```python
from build123d import *

# Parameters (mm, degrees)
SKETCH1_R               = 25
BOSS_EXTRUDE1_DEPTH     = 5
SKETCH3_R               = 1
CUT_EXTRUDE2_DEPTH      = 6
SKETCH4_R               = 25
SKETCH4_R_2             = 20.666666667
BOSS_EXTRUDE2_DEPTH     = 12
SKETCH2_R               = 1.3
CUT_EXTRUDE1_DEPTH      = 13
CUT_EXTRUDE1_DEPTH_BACK = 6
CUT_EXTRUDE3_DEPTH      = 6
CUT_EXTRUDE5_DEPTH      = 13
SKETCH8_R               = 2.3
SKETCH8_R_2             = 1.3
BOSS_EXTRUDE3_DEPTH     = 12


with BuildPart() as part:
    # Sketch1 → Boss-Extrude1 (new body)
    with BuildSketch(Plane(origin=(0, 0, 0), x_dir=(0, 0, -1), z_dir=(1, 0, 0))):
        Circle(SKETCH1_R)
    extrude(amount=BOSS_EXTRUDE1_DEPTH)

    # Sketch3 → Cut-Extrude2 (cut, through all)
    with BuildSketch(Plane.ZY):
        with Locations((-13.14, 13.14)):
            Circle(SKETCH3_R)
        with Locations((13.14, 13.14)):
            Circle(SKETCH3_R)
        with Locations((13.14, -13.14)):
            Circle(SKETCH3_R)
        with Locations((-13.14, -13.14)):
            Circle(SKETCH3_R)
    extrude(amount=-CUT_EXTRUDE2_DEPTH, mode=Mode.SUBTRACT)

    # Sketch4 → Boss-Extrude2 (add)
    with BuildSketch(Plane(origin=(5, 0, 0), x_dir=(0, 0, -1), z_dir=(1, 0, 0))):
        Circle(SKETCH4_R)
        Circle(SKETCH4_R_2, mode=Mode.SUBTRACT)
    extrude(amount=BOSS_EXTRUDE2_DEPTH)

    # Sketch2 → Cut-Extrude1 (cut, two sides)
    with BuildSketch(Plane(origin=(5, 0, 0), x_dir=(0, 0, -1), z_dir=(1, 0, 0))) as cut_extrude1_sk:
        with Locations((0, 21.5)):
            Circle(SKETCH2_R)
        with Locations((21.5, 0)):
            Circle(SKETCH2_R)
        with Locations((0, -21.5)):
            Circle(SKETCH2_R)
        with Locations((-21.5, 0)):
            Circle(SKETCH2_R)
    extrude(amount=CUT_EXTRUDE1_DEPTH, mode=Mode.SUBTRACT)
    extrude(cut_extrude1_sk.sketch, amount=-CUT_EXTRUDE1_DEPTH_BACK, mode=Mode.SUBTRACT)

    # Sketch5 → Cut-Extrude3 (cut, through all)
    with BuildSketch(Plane(origin=(5, 0, 0), x_dir=(0, 0, -1), z_dir=(1, 0, 0))):
        with BuildLine():
            Line((9.75, -8.14), (-9.75, -8.14))
            ThreePointArc((-9.75, -8.14), (-10.457106781, -8.432893219), (-10.75, -9.14))
            Line((-10.75, -9.14), (-10.75, -17.14))
            ThreePointArc((-10.75, -17.14), (-10.457106781, -17.847106781), (-9.75, -18.14))
            Line((-9.75, -18.14), (9.75, -18.14))
            ThreePointArc((9.75, -18.14), (10.457106781, -17.847106781), (10.75, -17.14))
            Line((10.75, -17.14), (10.75, -12.14))
            ThreePointArc((10.75, -12.14), (11.042893219, -11.432893219), (11.75, -11.14))
            Line((11.75, -11.14), (14.53, -11.14))
            ThreePointArc((14.53, -11.14), (15.237106781, -10.847106781), (15.53, -10.14))
            Line((15.53, -10.14), (15.53, -4.14))
            ThreePointArc((15.53, -4.14), (15.237106781, -3.432893219), (14.53, -3.14))
            Line((14.53, -3.14), (11.75, -3.14))
            ThreePointArc((11.75, -3.14), (11.042893219, -3.432893219), (10.75, -4.14))
            Line((10.75, -4.14), (10.75, -7.14))
            ThreePointArc((10.75, -7.14), (10.457106781, -7.847106781), (9.75, -8.14))
        make_face()
    extrude(amount=-CUT_EXTRUDE3_DEPTH, mode=Mode.SUBTRACT)

    # Sketch7 → Cut-Extrude5 (cut, through all)
    with BuildSketch(Plane(origin=(5, 0, 0), x_dir=(0, 0, -1), z_dir=(1, 0, 0))):
        with BuildLine():
            Line((-10.665126266, 15.614873734), (0, 4.949747468))
            Line((0, 4.949747468), (10.665126266, 15.614873734))
            ThreePointArc((10.665126266, 15.614873734), (15.614873734, 15.614873734), (15.614873734, 10.665126266))
            Line((15.614873734, 10.665126266), (4.949747468, 0))
            Line((4.949747468, 0), (15.614873734, -10.665126266))
            ThreePointArc((15.614873734, -10.665126266), (15.614873734, -15.614873734), (10.665126266, -15.614873734))
            Line((10.665126266, -15.614873734), (0, -4.949747468))
            Line((0, -4.949747468), (-10.665126266, -15.614873734))
            ThreePointArc((-10.665126266, -15.614873734), (-15.614873734, -15.614873734), (-15.614873734, -10.665126266))
            Line((-15.614873734, -10.665126266), (-4.949747468, 0))
            Line((-4.949747468, 0), (-15.614873734, 10.665126266))
            ThreePointArc((-15.614873734, 10.665126266), (-15.614873734, 15.614873734), (-10.665126266, 15.614873734))
        make_face()
    extrude(amount=CUT_EXTRUDE5_DEPTH, mode=Mode.SUBTRACT)

    # Sketch8 → Boss-Extrude3 (add)
    with BuildSketch(Plane(origin=(5, 0, 0), x_dir=(0, 0, -1), z_dir=(1, 0, 0))):
        with Locations((0, -21.5)):
            Circle(SKETCH8_R)
        with Locations((0, -21.5)):
            Circle(SKETCH8_R_2, mode=Mode.SUBTRACT)
        with Locations((-21.5, 0)):
            Circle(SKETCH8_R)
        with Locations((-21.5, 0)):
            Circle(SKETCH8_R_2, mode=Mode.SUBTRACT)
        with Locations((0, 21.5)):
            Circle(SKETCH8_R)
        with Locations((0, 21.5)):
            Circle(SKETCH8_R_2, mode=Mode.SUBTRACT)
        with Locations((21.5, 0)):
            Circle(SKETCH8_R)
        with Locations((21.5, 0)):
            Circle(SKETCH8_R_2, mode=Mode.SUBTRACT)
    extrude(amount=BOSS_EXTRUDE3_DEPTH)


solid = part.part
```
For this review, take the finished solid that the model builds, in its own axes (mm). A direction names the side the tool comes from. Round coordinates to 2 decimals unless told otherwise and drop trailing zeros. Write each loop counter-clockwise with the first axis right and the second up, starting at its lowest first coordinate (ties: lowest second). Pieces come first, ordered by that corner, then holes.
1) Take a section at B-B on z = 0. Give the boundary of the cut face in (x, y), then the cut area to 3 significant figures.
Answer below:
outline: (0, -25) - (17, -25) - (17, -22.8) - (0, -22.8) - close; (0, -20.2) - (17, -20.2) - (17, -19.2) - (5, -19.2) - (5, -18.14) - (0, -18.14) - close; (0, -8.14) - (5, -8.14) - (5, 19.2) - (17, 19.2) - (17, 20.2) - (0, 20.2) - close; (0, 22.8) - (17, 22.8) - (17, 25) - (0, 25) - close
area: 251 mm2
2) Take a section at A-A on x = 13.75. Give the boundary of the cut face in (y, z).
Answer below:
outline: circle Ø50 at (0, 0); hole circle Ø2.6 at (-21.5, 0); hole (-20.56, -2.1) arc R20.67 ccw to (-16.55, -12.37) arc R3.5 ccw to (-12.37, -16.55) arc R20.67 ccw to (-2.1, -20.56) arc R2.3 cw to (2.1, -20.56) arc R20.67 ccw to (12.37, -16.55) arc R3.5 ccw to (16.55, -12.37) arc R20.67 ccw to (20.56, -2.1) arc R2.3 cw to (20.56, 2.1) arc R20.67 ccw to (16.55, 12.37) arc R3.5 ccw to (12.37, 16.55) arc R20.67 ccw to (2.1, 20.56) arc R2.3 cw to (-2.1, 20.56) arc R20.67 ccw to (-12.37, 16.55) arc R3.5 ccw to (-16.55, 12.37) arc R20.67 ccw to (-20.56, 2.1) arc R2.3 cw to start; hole circle Ø2.6 at (0, -21.5); hole circle Ø2.6 at (0, 21.5); hole circle Ø2.6 at (21.5, 0)
3) Mouldability with a two-part tool opening along Z and no side actions: class faces 3 (the face through (0, 0, 0)), 4 (the face through (10.916, 19.283, 7.435)) as +Z half, -Z half, draft (parallel to the pull), parting line (faces both ways), or undercut.
Answer below:
face 3: draft
face 4: undercut
4) For line 1 along Y through (x, z) = (3.55, 0); line 2 along Y through (x, z) = (10.5, -0.5) (3 decimals); line 3 along Y through (x, z) = (11.75, 7.5), list the stretches that pass through material, from the lowest coordinate up.
Answer below:
line 1: y = -25 to -22.8, -20.2 to -18.14, -8.14 to 20.2, 22.8 to 25
line 2: y = -24.995 to -22.7, -20.3 to -19.255, 19.255 to 20.3, 22.7 to 24.995
line 3: y = -23.85 to -19.26, 19.26 to 23.85
5) Take a section at C-C on y = 13.14. Give the boundary of the cut face in (x, z).
Answer below:
outline: (0, -21.27) - (17, -21.27) - (17, -16.64) - (5, -16.64) - (5, -14.14) - (0, -14.14) - close; (0, -12.14) - (5, -12.14) - (5, 12.14) - (0, 12.14) - close; (0, 14.14) - (5, 14.14) - (5, 16.64) - (17, 16.64) - (17, 21.27) - (0, 21.27) - close
6) Take a section at D-D on z = 21.5. Give the boundary of the cut face in (x, y).
Answer below:
outline: (0, -12.76) - (17, -12.76) - (17, -1.3) - (0, -1.3) - close; (0, 1.3) - (17, 1.3) - (17, 12.76) - (0, 12.76) - close
7) Insertion check: pin 1 Ø3 at (x, z) = (3.5, -14) entering from -Y; pin 2 Ø10 at (x, z) = (7, -0.5) entering from +Y; pin 3 Ø1.6 at (y, z) = (0, 21.5) entering from -X; pin 4 Ø1 at (x, z) = (12, 11.5) entering from -Y. Each pin has a flat end and moves straight along its axis. Give the tip position at first contact, or say it passes through.
Answer below:
pin 1: stops at y = -21.65
pin 2: stops at y = 25
pin 3: passes through
pin 4: stops at y = -22.45
8) Machinability: for faces 1 (the face through (3, -15, -10.75)), 2 (the face through (10.92, 15.58, 15.65)), which of the approach directions +Z, -Z, +X, -X, +Y, -Y give a long, thin tool a straight path to every point of the face, cutting with its end or side? Answer none if there is none.
Answer below:
face 1: +X, -X
face 2: +X
